Design review of the part built by this model. Coordinates are the model's own, in mm. Face numbers are marked on the shaded views. A direction names the side the tool comes from. Round coordinates to 2 decimals unless told otherwise and drop trailing zeros. Order: outer loops, then holes, each group sorted by start corner. A loop starts at its lowest first (then second) coordinate and runs counter-clockwise, first axis right, second up. Notation, with made-up numbers: (-15, -11.5) - (35, -11.5) arc R19 ccw to (35, -7.5) - close; hole circle Ø3 at (-38, 79.25). An arc over 180 degrees is marked (long way). Write item = value, one per line.
from build123d import *

# Parameters (mm, degrees)
F1_DEPTH = 300
F2_W     = 70
F2_H     = 80
F3_DEPTH = 25
F4_DEPTH = 25
F5_DEPTH = 25
F6_R     = 2.5
F7_DEPTH = 25


with BuildPart() as f1:
    # F0 (on Front) → F1 (new body)
    with BuildSketch(Plane.XZ):
        with BuildLine():
            Line((75, 38.914216), (75, 52.5))
            Line((75, 52.5), (74, 52.5))
            Line((74, 52.5), (74, 38.875))
            ThreePointArc((74, 38.875), (73.361451, 36.706903), (71.649678, 35.231024))
            ThreePointArc((71.649678, 35.231024), (60.8185, 29.988223), (54.643786, 19.659898))
            Line((54.643786, 19.659898), (43.416317, -24.63337))
            ThreePointArc((43.416317, -24.63337), (41.948954, -27.705545), (39.413109, -29.977308))
            Line((39.413109, -29.977308), (26.950339, -37.332837))
            ThreePointArc((26.950339, -37.332837), (24.789532, -39.524934), (24, -42.5))
            Line((24, -42.5), (24, -51.5))
            Line((24, -51.5), (-73, -51.5))
            ThreePointArc((-73, -51.5), (-73.707107, -51.207107), (-74, -50.5))
            Line((-74, -50.5), (-74, 52.5))
            Line((-74, 52.5), (-75, 52.5))
            Line((-75, 52.5), (-75, -50.5))
            ThreePointArc((-75, -50.5), (-74.414214, -51.914214), (-73, -52.5))
            Line((-73, -52.5), (25, -52.5))
            Line((25, -52.5), (25, -42.5))
            ThreePointArc((25, -42.5), (25.657943, -40.020778), (27.458616, -38.194031))
            Line((27.458616, -38.194031), (39.921386, -30.838502))
            ThreePointArc((39.921386, -30.838502), (42.749295, -28.305091), (44.385661, -24.87908))
            Line((44.385661, -24.87908), (55.613129, 19.414189))
            ThreePointArc((55.613129, 19.414189), (61.539869, 29.29273), (71.932405, 34.263346))
            ThreePointArc((71.932405, 34.263346), (74.173992, 36.121942), (75, 38.914216))
        make_face()
    extrude(amount=F1_DEPTH)

    # F2 (on face) → F3 (cut)
    with BuildSketch(Plane(origin=(0, 0, -52.5), x_dir=(1, 0, 0), z_dir=(0, 0, -1))):
        with Locations((-24, 150)):
            Rectangle(F2_W, F2_H)
    extrude(amount=-F3_DEPTH, mode=Mode.SUBTRACT)

    # F2 (on face) → F4 (cut)
    with BuildSketch(Plane(origin=(0, 0, -52.5), x_dir=(1, 0, 0), z_dir=(0, 0, -1))):
        with Locations((-24, 150)):
            Rectangle(F2_W, F2_H)
    extrude(amount=-F4_DEPTH, mode=Mode.SUBTRACT)

    # F2 (on face) → F5 (cut)
    with BuildSketch(Plane(origin=(0, 0, -52.5), x_dir=(1, 0, 0), z_dir=(0, 0, -1))):
        with Locations((-24, 150)):
            Rectangle(F2_W, F2_H)
    extrude(amount=-F5_DEPTH, mode=Mode.SUBTRACT)

    # F6 (on face) → F7 (cut)
    with BuildSketch(Plane(origin=(0, 0, -52.5), x_dir=(1, 0, 0), z_dir=(0, 0, -1))):
        with Locations((13, 268)):
            Circle(F6_R)
    extrude(amount=-F7_DEPTH, mode=Mode.SUBTRACT)


solid = f1.part
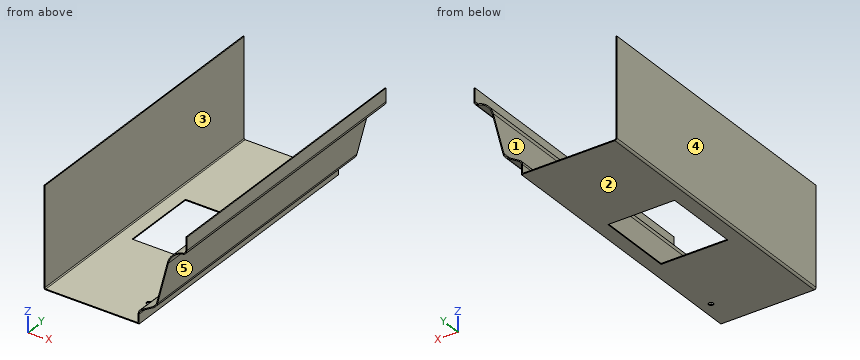
1) We need section C-C on y = -256.5. Write out the cut boundary in (x, z) (1 decimal).
Findings:
outline = (-75, -50.5) arc R2 ccw to (-73, -52.5) - (25, -52.5) - (25, -42.5) arc R5 cw to (27.5, -38.2) - (39.9, -30.8) arc R9.7 ccw to (44.4, -24.9) - (55.6, 19.4) arc R20 cw to (71.9, 34.3) arc R5 ccw to (75, 38.9) - (75, 52.5) - (74, 52.5) - (74, 38.9) arc R4 cw to (71.6, 35.2) arc R21 ccw to (54.6, 19.7) - (43.4, -24.6) arc R8.7 cw to (39.4, -30) - (27, -37.3) arc R6 ccw to (24, -42.5) - (24, -51.5) - (-73, -51.5) arc R1 cw to (-74, -50.5) - (-74, 52.5) - (-75, 52.5) - close
2) We need section D-D on z = 12. Write out the cut boundary in (x, y).
Findings:
outline = (-75, -300) - (-74, -300) - (-74, 0) - (-75, 0) - close; (52.7, -300) - (53.73, -300) - (53.73, 0) - (52.7, 0) - close
3) Clearance check with flat-ended pins moving along their axes: pin 1 Ø0.8 at (y, z) = (-167, -52) entering from +X; pin 2 Ø0.8 at (y, z) = (-161, -52) entering from -X; pin 3 Ø6 at (y, z) = (-248, -9.5) entering from +X. State where each tip first meets the part, or that it passes through.
Findings:
pin_1 = 25
pin_2 = -74.67
pin_3 = 49.04
4) The part is to be moulded in two halves that separate along X. For the marked faces 3, 4 and 5, say which applies: released by +X, released by -X, zero draft, split by the parting line, or undercut.
Findings:
face_3 = undercut
face_4 = released by -X
face_5 = released by +X
5) For the marked faces 1 and 2, list the 3-axis set-ups (+Z, -Z, +X, -X, +Y, -Y) from which the entire face can be reached by the end or side of a thin tool; tool diameter is ignored.
Findings:
face_1 = +Z, +Y, -Y
face_2 = -Z, +X, -X, +Y, -Y
6) We need section A-A on x = -22.5. Write out the cut boundary in (y, z).
Findings:
outline = (-300, -52.5) - (-190, -52.5) - (-190, -51.5) - (-300, -51.5) - close; (-110, -52.5) - (0, -52.5) - (0, -51.5) - (-110, -51.5) - close
7) To check wall thickness, follow L1, parallel to Y at x = 13, z = -52; L2, parallel to X at y = -255.5, z = -46.5; L3, parallel to X at y = -268, z = -52.2. State the ranges of each line that lie inside material, in increasing order. Write a range as from..to.
Findings:
L1 = -300..-270.5, -265.5..0
L2 = -75..-74, 24..25
L3 = -74.05..10.5, 15.5..25
8) We need section B-B on y = -154.5. Write out the cut boundary in (x, z) (1 decimal), and give its area (3 significant figures).
Findings:
outline = (-75, -50.5) arc R2 ccw to (-73, -52.5) - (-59, -52.5) - (-59, -51.5) - (-73, -51.5) arc R1 cw to (-74, -50.5) - (-74, 52.5) - (-75, 52.5) - close; (11, -52.5) - (25, -52.5) - (25, -42.5) arc R5 cw to (27.5, -38.2) - (39.9, -30.8) arc R9.7 ccw to (44.4, -24.9) - (55.6, 19.4) arc R20 cw to (71.9, 34.3) arc R5 ccw to (75, 38.9) - (75, 52.5) - (74, 52.5) - (74, 38.9) arc R4 cw to (71.6, 35.2) arc R21 ccw to (54.6, 19.7) - (43.4, -24.6) arc R8.7 cw to (39.4, -30) - (27, -37.3) arc R6 ccw to (24, -42.5) - (24, -51.5) - (11, -51.5) - close
area = 258 mm^2
